```python
from build123d import *

# Parameters (mm, degrees)
SKETCH_1_W                = 32
SKETCH_1_H                = 35
EXTRUDE_1_DEPTH           = 10.75
SKETCH_3_W                = 3
SKETCH_3_H                = 2.25
CUT_EXTRUDE_1_DEPTH       = 49.62676732
SKETCH_6_R                = 4.5
CUT_EXTRUDE_4_DEPTH       = 2.25
EXTRUDE_2_DEPTH           = 8.5
SKETCH_10_R               = 1.25
CUT_EXTRUDE_5_DEPTH       = 74.243173743
CUT_EXTRUDE_8_DEPTH       = 4
SKETCH_13_W               = 2
SKETCH_13_H               = 2.25
EXTRUDE_3_DEPTH           = 15
SKETCH_14_R               = 3
CUT_EXTRUDE_9_DEPTH       = 73.946898495
CUT_EXTRUDE_10_DEPTH      = 68.797953509
CUT_EXTRUDE_10_DEPTH_BACK = 68.797953509
SKETCH_15_W               = 8.485281374
SKETCH_15_H               = 2.25


with BuildPart() as part:
    # Эскиз1 → Бобышка-Вытянуть1 (new body)
    with BuildSketch(Plane(origin=(0, 0, 0), x_dir=(1, 0, 0), z_dir=(0, 1, 0))):
        with Locations((16, 17.5)):
            Rectangle(SKETCH_1_W, SKETCH_1_H)
    extrude(amount=EXTRUDE_1_DEPTH)

    # Эскиз3 → Вырез-Вытянуть1 (cut, through all)
    with BuildSketch(Plane.XY):
        with Locations((16, 1.125)):
            Rectangle(SKETCH_3_W, SKETCH_3_H)
        with Locations((21, 1.125)):
            Rectangle(SKETCH_3_W, SKETCH_3_H)
        with Locations((26, 1.125)):
            Rectangle(SKETCH_3_W, SKETCH_3_H)
        with Locations((31, 1.125)):
            Rectangle(SKETCH_3_W, SKETCH_3_H)
        with Locations((11, 1.125)):
            Rectangle(SKETCH_3_W, SKETCH_3_H)
        with Locations((6, 1.125)):
            Rectangle(SKETCH_3_W, SKETCH_3_H)
        with Locations((1, 1.125)):
            Rectangle(SKETCH_3_W, SKETCH_3_H)
    extrude(amount=-CUT_EXTRUDE_1_DEPTH, mode=Mode.SUBTRACT)

    # Эскиз6 → Вырез-Вытянуть4 (cut)
    with BuildSketch(Plane.XZ):
        with Locations((16, -17.5)):
            Circle(SKETCH_6_R)
    extrude(amount=-CUT_EXTRUDE_4_DEPTH, mode=Mode.SUBTRACT)

    # Эскиз7 → Бобышка-Вытянуть2 (add)
    with BuildSketch(Plane(origin=(0, 10.75, 0), x_dir=(1, 0, 0), z_dir=(0, 1, 0))):
        with BuildLine():
            Line((0, 0), (0, -25))
            ThreePointArc((0, -25), (1.464466094, -28.535533906), (5, -30))
            Line((5, -30), (27, -30))
            ThreePointArc((27, -30), (30.535533906, -28.535533906), (32, -25))
            Line((32, -25), (32, 0))
            Line((32, 0), (0, 0))
        make_face()
        with BuildLine():
            Line((5.75, -21.25), (26.25, -21.25))
            ThreePointArc((26.25, -21.25), (28.5, -23.5), (26.25, -25.75))
            Line((26.25, -25.75), (5.75, -25.75))
            ThreePointArc((5.75, -25.75), (3.5, -23.5), (5.75, -21.25))
        make_face(mode=Mode.SUBTRACT)
    extrude_2 = extrude(amount=-EXTRUDE_2_DEPTH)

    # Зеркальное отражение1: Бобышка-Вытянуть2 across plane
    add(extrude_2.mirror(Plane.XY.offset(-17.5)))

    # Эскиз10 → Вырез-Вытянуть5 (cut, through all)
    with BuildSketch(Plane(origin=(0, 10.75, 0), x_dir=(1, 0, 0), z_dir=(0, 1, 0))):
        with Locations(Location((4, 29.5, 0), (0, 0, 270))):
            Circle(SKETCH_10_R)
        with Locations(Location((4, 5.5, 0), (0, 0, 270))):
            Circle(SKETCH_10_R)
        with Locations(Location((28, 5.5, 0), (0, 0, 270))):
            Circle(SKETCH_10_R)
        with Locations(Location((28, 29.5, 0), (0, 0, 270))):
            Circle(SKETCH_10_R)
    extrude(amount=-CUT_EXTRUDE_5_DEPTH, mode=Mode.SUBTRACT)

    # Эскиз11 → Вырез-Вытянуть8 (cut)
    with BuildSketch(Plane.XZ.offset(-2.25)):
        Polygon((25.690598923, -5.5), (26.845299462, -7.5), (29.154700538, -7.5), (30.309401077, -5.5), (29.154700538, -3.5), (26.845299462, -3.5), align=None)
        Polygon((6.309401077, -5.5), (5.154700538, -3.5), (2.845299462, -3.5), (1.690598923, -5.5), (2.845299462, -7.5), (5.154700538, -7.5), align=None)
        Polygon((6.309401077, -29.5), (5.154700538, -27.5), (2.845299462, -27.5), (1.690598923, -29.5), (2.845299462, -31.5), (5.154700538, -31.5), align=None)
        Polygon((25.690598923, -29.5), (26.845299462, -31.5), (29.154700538, -31.5), (30.309401077, -29.5), (29.154700538, -27.5), (26.845299462, -27.5), align=None)
    extrude(amount=-CUT_EXTRUDE_8_DEPTH, mode=Mode.SUBTRACT)

    # Эскиз13 → Бобышка-Вытянуть3 (add)
    with BuildSketch(Plane.XY):
        with Locations((28.5, 1.125)):
            Rectangle(SKETCH_13_W, SKETCH_13_H)
        with Locations((23.5, 1.125)):
            Rectangle(SKETCH_13_W, SKETCH_13_H)
        with Locations((18.5, 1.125)):
            Rectangle(SKETCH_13_W, SKETCH_13_H)
        with Locations((13.5, 1.125)):
            Rectangle(SKETCH_13_W, SKETCH_13_H)
        with Locations((8.5, 1.125)):
            Rectangle(SKETCH_13_W, SKETCH_13_H)
        with Locations((3.5, 1.125)):
            Rectangle(SKETCH_13_W, SKETCH_13_H)
    extrude_3 = extrude(amount=EXTRUDE_3_DEPTH)

    # Зеркальное отражение2: Бобышка-Вытянуть3 across plane
    add(extrude_3.mirror(Plane.XY.offset(-17.5)))

    # Эскиз14 → Вырез-Вытянуть9 (cut, through all)
    with BuildSketch(Plane.XZ.offset(-2.25)):
        with Locations((28, -5.5)):
            Circle(SKETCH_14_R)
        with Locations((28, -29.5)):
            Circle(SKETCH_14_R)
        with Locations((4, -29.5)):
            Circle(SKETCH_14_R)
        with Locations((4, -5.5)):
            Circle(SKETCH_14_R)
    extrude(amount=CUT_EXTRUDE_9_DEPTH, mode=Mode.SUBTRACT)

    # Эскиз15 → Вырез-Вытянуть10 (cut, two sides: drawn at the far end of the back side and taken through both)
    with BuildSketch(Plane(origin=(16, 0, 0), x_dir=(0, 0, -1), z_dir=(1, 0, 0)).offset(-CUT_EXTRUDE_10_DEPTH_BACK)):
        with Locations((17.5, 1.125)):
            Rectangle(SKETCH_15_W, SKETCH_15_H)
    extrude(amount=CUT_EXTRUDE_10_DEPTH + CUT_EXTRUDE_10_DEPTH_BACK, mode=Mode.SUBTRACT)


solid = part.part
```
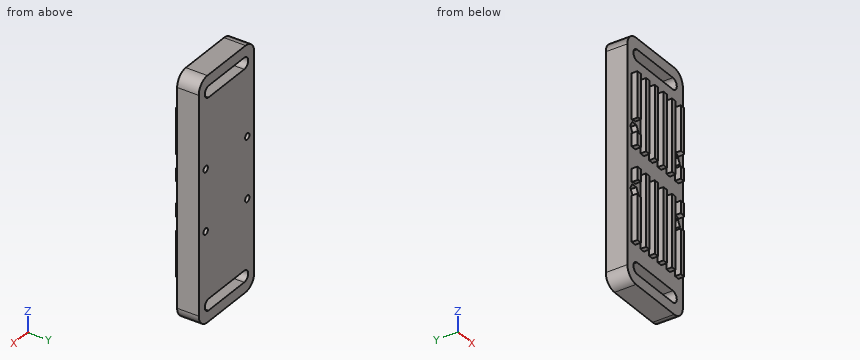
The model under review builds one solid part; all positions refer to its coordinate system, in mm. Round coordinates to 2 decimals unless told otherwise and drop trailing zeros. Loops run counter-clockwise (first coordinate to the right, second up) from the corner with the lowest first, then second, coordinate; pieces in that order, holes last. Notation, with made-up numbers: (86, 39) - (104, 39) arc R21 ccw to (104, 62) - close; hole circle Ø3 at (-8.5, 89). An arc over 180 degrees is marked (long way). Write each question's results on one line, items separated by ' | '. Start each with the question number.
Q1. Take a section at B-B on z = -58.5. Give the boundary of the cut face in (x, y), plus the area to 3 significant figures.
Q2. Take a section at A-A on y = 7.5. Give the boundary of the cut face in (x, z), plus the area to 3 significant figures.
Q3. Take a section at C-C on y = 1.25. Give the number of separate pieces and of enclosed holes in the cut face, plus the area to 3 significant figures.
Q4. Wall thickness on line 1 along Z through (x, y) = (22.5, 5.5); line 2 along X through (y, z) = (8.05, -5.5); line 3 along Z through (x, y) = (9, 0.75): over which ranges is each line inside the solid? List them lowest first. Write a range as [from, to].
Q5. Insertion check: P1, Ø2, axis at x = 3, y = 1.5, coming from the +Z side; P2, Ø1.2, axis at x = 4, y = 3.5, coming from the +Z side; P3, Ø1.2, axis at x = 28.5, y = 3.5, coming from the -Z side. Each pin has a flat end and moves straight along its axis. Give the tip position at first contact, or say it passes through.
Q6. Take a section at D-D on z = 13.5. Give the boundary of the cut face in (x, y).
Data:
1) outline: (0, 2.25) - (3.5, 2.25) - (3.5, 10.75) - (0, 10.75) - close; (28.5, 2.25) - (32, 2.25) - (32, 10.75) - (28.5, 10.75) - close | area: 59.5 mm²
2) outline: (0, -60) arc R5 ccw to (5, -65) - (27, -65) arc R5 ccw to (32, -60) - (32, 25) arc R5 ccw to (27, 30) - (5, 30) arc R5 ccw to (0, 25) - close; hole circle Ø2.5 at (4, -29.5); hole circle Ø2.5 at (4, -5.5); hole (5.75, -60.75) - (26.25, -60.75) arc R2.25 ccw to (26.25, -56.25) - (5.75, -56.25) arc R2.25 ccw to start; hole (5.75, 21.25) - (26.25, 21.25) arc R2.25 ccw to (26.25, 25.75) - (5.75, 25.75) arc R2.25 ccw to start; hole circle Ø2.5 at (28, -29.5); hole circle Ø2.5 at (28, -5.5) | area: 2,780 mm²
3) separate pieces: 16 | enclosed holes: 0 | area: 632 mm²
4) line 1: z = [-65, -60.75], [-56.25, 21.25], [25.75, 30] | line 2: x = [0, 2.75], [5.25, 26.75], [29.25, 32] | line 3: z = [-50, -21.74], [-13.26, 15]
5) P1: stops at z = 29.82 | P2: stops at z = 29.98 | P3: stops at z = -64.92
6) outline: (0, 2.25) - (2.5, 2.25) - (2.5, 0) - (4.5, 0) - (4.5, 2.25) - (7.5, 2.25) - (7.5, 0) - (9.5, 0) - (9.5, 2.25) - (12.5, 2.25) - (12.5, 0) - (14.5, 0) - (14.5, 2.25) - (17.5, 2.25) - (17.5, 0) - (19.5, 0) - (19.5, 2.25) - (22.5, 2.25) - (22.5, 0) - (24.5, 0) - (24.5, 2.25) - (27.5, 2.25) - (27.5, 0) - (29.5, 0) - (29.5, 2.25) - (32, 2.25) - (32, 10.75) - (0, 10.75) - close
